Input: part model. Units: mm. Frame: model coordinates. A direction names the side the tool comes from. Round coordinates to 2 decimals unless told otherwise and drop trailing zeros. Order: outer loops, then holes, each group sorted by start corner. A loop starts at its lowest first (then second) coordinate and runs counter-clockwise, first axis right, second up. Notation, with made-up numbers: (-36.75, -38.5) -> (11.25, -38.5) arc R24 ccw to (11.25, -18.5) -> close; hole circle Ø1 at (-15.5, 38.5). An arc over 180 degrees is marked (long way). Use a Markdown table: item, result.
from build123d import *

# Parameters (mm, degrees)
F3_D = 3.175
F4_R = 3.175
F5_R = 3.175


with BuildPart() as f1:
    # F0 (on Front) → F1 (revolve)
    with BuildSketch(Plane.XZ):
        Polygon((-63.5, 3.175), (-63.5, 0), (-47.625, 0), (-47.625, 28.575), (-50.8, 28.575), (-50.8, 3.175), align=None)
    revolve(axis=Axis((0, 0, 11.316922), (0, 0, -1)))

    # F3 (through all)
    with Locations(Plane(origin=(0, 0, 0), x_dir=(1, 0, 0), z_dir=(0, 0, -1))):
        with Locations((-57.15, 0), (0, 57.15), (57.15, 0), (0, -57.15)):
            Hole(F3_D / 2)

    # F4
    f4_edges = [f1.edges().sort_by_distance(p)[0] for p in [
        (47.625, 0, 0),
    ]]
    fillet(f4_edges, radius=F4_R)

    # F5
    f5_edges = [f1.edges().sort_by_distance(p)[0] for p in [
        (50.8, 0, 3.175),
    ]]
    fillet(f5_edges, radius=F5_R)


solid = f1.part
1) Cut plane C-C on z = 14.25. Return loops of the section in (x, y) (3 decimals).
Answer key:
| item | result |
|---|---|
| outline | circle Ø101.6 at (0, 0); hole circle Ø95.25 at (0, 0) |
2) Contact query for flat-ended pins moving along their axis: P1, Ø4, axis at x = 0, y = 57.15, coming from the +Z side (3 decimals); P2, Ø2.5, axis at x = 57.15, y = 0, coming from the +Z side; P3, Ø12, axis at x = -5, y = -42.5, coming from the -Z side; P4, Ø6, axis at y = -25.5, z = 22.5, coming from the +X side. Output: stop coordinate, or through.
Answer key:
| item | result |
|---|---|
| P1 | stops at z = 3.175 |
| P2 | passes through |
| P3 | stops at z = 0.71 |
| P4 | stops at x = 45.55 |
3) Ray query, probe 1 along Y at (x, z) = (0, 10.25) (3 decimals); probe 2 along Y at (x, z) = (0, 0.85); probe 3 along Z at (x, y) = (-7, -57) (3 decimals). Return the intervals inside material, ascending.
Answer key:
| item | result |
|---|---|
| probe 1 | y = -50.8 to -47.625, 47.625 to 50.8 |
| probe 2 | y = -63.5 to -58.74, -55.56 to -48.64, 48.64 to 55.56, 58.74 to 63.5 |
| probe 3 | z = 0 to 3.175 |
4) Set-up query: faces 1 (the face through (0.34, -55.6, 1.61)), 2 (the face through (11.012, -49.592, 17.307)). Return all of +Z, -Z, +X, -X, +Y, -Y with unobstructed straight access to the full face (end or side cutting, diameter ignored); none if empty.
Answer key:
| item | result |
|---|---|
| face 1 | +Z, -Z |
| face 2 | +Z |
5) Cut plane B-B on y = 57.15. Return loops of the section in (x, z) (1 decimal), and give its area (3 significant figures).
Answer key:
| item | result |
|---|---|
| outline | (-27.7, 0) -> (-1.6, 0) -> (-1.6, 3.2) -> (-27.7, 3.2) -> close; (1.6, 0) -> (27.7, 0) -> (27.7, 3.2) -> (1.6, 3.2) -> close |
| area | 166 mm^2 |
6) Cut plane A-A on x = 0. State how many separate pieces and enclosed holes the cut face has, and give its area (3 significant figures).
Answer key:
| item | result |
|---|---|
| separate pieces | 4 |
| enclosed holes | 0 |
| area | 242 mm^2 |
7) Draft query along X for faces 3 (the face through (-58.664, -0.477, 1.61)), 4 (the face through (-15.3, 45.4, 28.575)), 5 (the face through (13.77, -61.99, 1.57)). Return one class per face: released by +X, released by -X, zero draft, split by the parting line, or undercut.
Answer key:
| item | result |
|---|---|
| face 3 | undercut |
| face 4 | zero draft |
| face 5 | split by the parting line |
